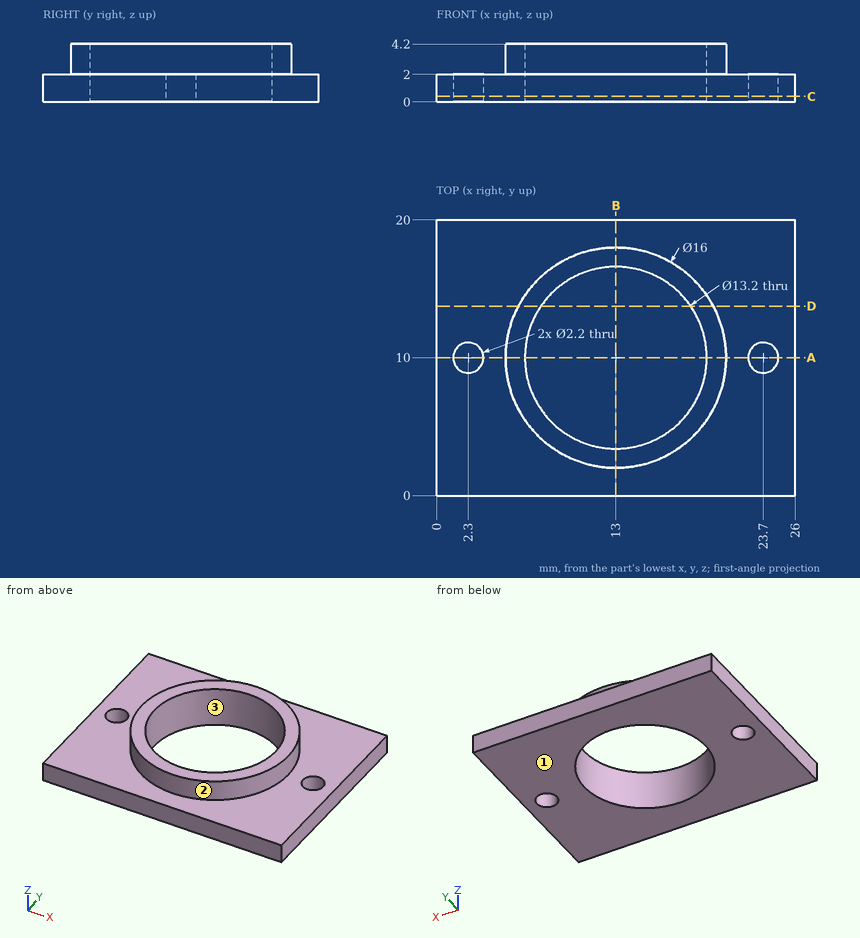
Geometry check sheet. Reference: drawing and pictorial views, mm from the part's lowest x, y, z. Coordinates: 2 decimals unless noted, no trailing zeros. Order: outer loops, then holes, each group sorted by start corner. A loop starts at its lowest first (then second) coordinate and runs counter-clockwise, first axis right, second up. Notation, with made-up numbers: (74.5, 33.5) - (100.5, 33.5) arc R26 ccw to (100.5, 60.5) - close; hole circle Ø6 at (76.25, 54). An arc over 180 degrees is marked (long way). Answer in a Markdown table with one row per item. Add a question column.
1) Release check for a two-part mould opening along X. For the marked faces 1, 2 and 3 record: +X half, -X half, draft (parallel to the pull), parting line (faces both ways), or undercut.
2) Gauge pin test, flat end, axial feed: P1, Ø1, axis at x = 18.5, y = 11.5, coming from the -Z side. Record the tip position at first contact, or that the pin passes through.
3) Cross-section at B-B, the plane x = 13. Record the cut outline in (y, z).
4) Cross-section at A-A, the plane y = 10. Record the cut outline in (x, z).
5) Cross-section at C-C, the plane z = 0.4. Record the cut outline in (x, y).
6) Material ranges on line 1 along Y through (x, z) = (2.3, 0.9); line 2 along Y through (x, z) = (13, 2.9); line 3 along Z through (x, y) = (18.75, 15.75), recorded low to high. Write a range as [from, to].
7) Cross-section at D-D, the plane y = 13.75. Record the cut outline in (x, z).
Check result:
| question | item | result |
|---|---|---|
| 1 | face 1 | draft |
| 1 | face 2 | parting line |
| 1 | face 3 | undercut |
| 2 | P1 | passes through |
| 3 | outline | (0, 0) - (3.4, 0) - (3.4, 4.2) - (2, 4.2) - (2, 2) - (0, 2) - close; (16.6, 0) - (20, 0) - (20, 2) - (18, 2) - (18, 4.2) - (16.6, 4.2) - close |
| 4 | outline | (0, 0) - (1.2, 0) - (1.2, 2) - (0, 2) - close; (3.4, 0) - (6.4, 0) - (6.4, 4.2) - (5, 4.2) - (5, 2) - (3.4, 2) - close; (19.6, 0) - (22.6, 0) - (22.6, 2) - (21, 2) - (21, 4.2) - (19.6, 4.2) - close; (24.8, 0) - (26, 0) - (26, 2) - (24.8, 2) - close |
| 5 | outline | (0, 0) - (26, 0) - (26, 20) - (0, 20) - close; hole circle Ø2.2 at (2.3, 10); hole circle Ø13.2 at (13, 10); hole circle Ø2.2 at (23.7, 10) |
| 6 | line 1 | y = [0, 8.9], [11.1, 20] |
| 6 | line 2 | y = [2, 3.4], [16.6, 18] |
| 6 | line 3 | z = [0, 2] |
| 7 | outline | (0, 0) - (7.57, 0) - (7.57, 4.2) - (5.93, 4.2) - (5.93, 2) - (0, 2) - close; (18.43, 0) - (26, 0) - (26, 2) - (20.07, 2) - (20.07, 4.2) - (18.43, 4.2) - close |
